Here's how the part is built. I have some questions about the finished solid (model axes, mm). A direction names the side the tool comes from. Coordinates: 2 decimals unless noted, no trailing zeros. Loops run counter-clockwise (first coordinate to the right, second up) from the corner with the lowest first, then second, coordinate; pieces in that order, holes last. Notation, with made-up numbers: (42, 27.25) -> (55, 27.25) arc R17 cw to (55, 31.25) -> close; hole circle Ø6 at (-37, 66.5). An arc over 180 degrees is marked (long way). Use CSV: the item, a comma, the result in double quotes. Start each with the question number.
from build123d import *

# Parameters (mm, degrees)
F0_W      = 40
F0_H      = 40
F1_DEPTH  = 16
F2_R      = 3.1
F3_DEPTH  = 14.7
F4_W      = 31.5
F4_H      = 31.5
F5_DEPTH  = 4
F8_DEPTH  = 7
F9_W      = 20
F9_H      = 20
F10_DEPTH = 3
F11_R     = 1.6
F12_DEPTH = 25
F14_R     = 4.8
F15_DEPTH = 1
F16_R     = 1.4
F17_DEPTH = 25


with BuildPart() as f1:
    # F0 (on Top) → F1 (new body)
    with BuildSketch(Plane.XY):
        Rectangle(F0_W, F0_H)
    extrude(amount=-F1_DEPTH)

    # F2 (on Top) → F3 (cut)
    with BuildSketch(Plane.XY):
        Circle(F2_R)
    extrude(amount=-F3_DEPTH, mode=Mode.SUBTRACT)

    # F4 (on Top) → F5 (cut)
    with BuildSketch(Plane.XY):
        with Locations((4.25, -4.25)):
            Rectangle(F4_W, F4_H)
    extrude(amount=-F5_DEPTH, mode=Mode.SUBTRACT)

    # F7 (on offset) → F8 (cut)
    with BuildSketch(Plane.XY.offset(-3.5)):
        Polygon((5.831176, -0.026889), (2.938874, 5.036502), (-2.892302, 5.063391), (-5.831176, 0.026889), (-2.938874, -5.036502), (2.892302, -5.063391), align=None)
    extrude(amount=-F8_DEPTH, mode=Mode.SUBTRACT)

    # F9 (on offset) → F10 (cut)
    with BuildSketch(Plane.XY.offset(-3.5)):
        with Locations((10, -10)):
            Rectangle(F9_W, F9_H)
    extrude(amount=-F10_DEPTH, mode=Mode.SUBTRACT)

    # F11 (on offset) → F12 (cut)
    with BuildSketch(Plane.XY.offset(-3.5)):
        with Locations((-8, 8)):
            Circle(F11_R)
        with Locations((12, 8)):
            Circle(F11_R)
        with Locations((-8, -12)):
            Circle(F11_R)
    extrude(amount=-F12_DEPTH, mode=Mode.SUBTRACT)

    # F14 (on offset) → F15 (cut)
    with BuildSketch(Plane.XY.offset(-16)):
        Circle(F14_R)
    extrude(amount=F15_DEPTH, mode=Mode.SUBTRACT)

    # F16 (on Top) → F17 (cut)
    with BuildSketch(Plane.XY):
        with Locations((-15.967699, 16)):
            Circle(F16_R)
        with Locations((16, 16)):
            Circle(F16_R)
        with Locations((-16, -16)):
            Circle(F16_R)
    extrude(amount=-F17_DEPTH, mode=Mode.SUBTRACT)


solid = f1.part
1) I want a section at D-D, the plane z = -6. Please give me the cut outline in (x, y).
2) I want a section at C-C, the plane x = 16. Please give me the cut outline in (y, z).
3) For P1, Ø6, axis at x = 0, y = 0, coming from the -Z side; P2, Ø7, axis at x = -0.5, y = 0, coming from the +Z side; P3, Ø3, axis at y = -13, z = -4.5, coming from the +X side, each with a flat end and sliding along its axis, tell me the tip position at first contact or that it passes through.
4) Thinking about a two-plate mould opening in Y: for faces 1 (the face through (13, 0, -5)), 2 (the face through (-5, 5, -16)), 3 (the face through (-4.34, 2.58, -7.2)), which applies, pulls with the +Y half, pulls with the -Y half, needs draft (parallel to the pull), parting line crosses it, or undercut?
5) I want a section at B-B, the plane x = -8. Please give me the cut outline in (y, z).
6) I want a section at A-A, the plane y = 16. Please give me the cut outline in (x, z).
7) Please list where these lines run through material, in increasing order: L1, parallel to Y at x = -8, z = -13.5; L2, parallel to Y at x = -16, z = -7.25; L3, parallel to Y at x = 0, z = -15.6. Write a range as [from, to].
8) Which directions (+Z, -Z, +X, -X, +Y, -Y) give clear straight access to the entire face, cutting with the end or side of a thin tool? Please do faces 4 (the face through (0, 0, -15)), 5 (the face through (3, 2, -10.5)), 6 (the face through (1, 6, -4)), 7 (the face through (10.4, 8.07, -9.92)).
Return value:
1,outline,"(-20, -20) -> (0, -20) -> (0, -5.05) -> (-2.94, -5.04) -> (-5.83, 0.03) -> (-2.89, 5.06) -> (2.94, 5.04) -> (5.82, 0) -> (20, 0) -> (20, 20) -> (-20, 20) -> close; hole circle Ø2.8 at (-16, -16); hole circle Ø2.8 at (-15.97, 16); hole circle Ø3.2 at (-8, -12); hole circle Ø3.2 at (-8, 8); hole circle Ø3.2 at (12, 8); hole circle Ø2.8 at (16, 16)"
2,outline,"(-20, -16) -> (14.6, -16) -> (14.6, 0) -> (11.5, 0) -> (11.5, -4) -> (0, -4) -> (0, -6.5) -> (-20, -6.5) -> close; (17.4, -16) -> (20, -16) -> (20, 0) -> (17.4, 0) -> close"
3,P1,"stops at z = -15"
3,P2,"stops at z = -10.5"
3,P3,"stops at x = 0"
4,face 1,"pulls with the -Y half"
4,face 2,"needs draft"
4,face 3,"undercut"
5,outline,"(-20, -16) -> (-13.6, -16) -> (-13.6, -4) -> (-20, -4) -> close; (-10.4, -16) -> (6.4, -16) -> (6.4, -4) -> (-10.4, -4) -> close; (9.6, -16) -> (20, -16) -> (20, 0) -> (11.5, 0) -> (11.5, -4) -> (9.6, -4) -> close"
6,outline,"(-20, -16) -> (-17.37, -16) -> (-17.37, 0) -> (-20, 0) -> close; (-14.57, -16) -> (14.6, -16) -> (14.6, 0) -> (-14.57, 0) -> close; (17.4, -16) -> (20, -16) -> (20, 0) -> (17.4, 0) -> close"
7,L1,"y = [-20, -13.6], [-10.4, 6.4], [9.6, 20]"
7,L2,"y = [-20, -17.4], [-14.6, 14.6], [17.4, 20]"
7,L3,"y = [-20, -4.8], [4.8, 20]"
8,face 4,"-Z"
8,face 5,"+Z"
8,face 6,"+Z, +X, -Y"
8,face 7,"+Z, -Z"
